Read the model definition and answer for the solid it produces. Units are mm, in the model's axes. Give positions to 0.01 mm unless a question says otherwise; leave off trailing zeros. Write each loop counter-clockwise with the first axis right and the second up, starting at its lowest first coordinate (ties: lowest second). Pieces come first, ordered by that corner, then holes. Notation, with made-up numbers: (34, 24) -> (93, 24) arc R34 cw to (93, 58) -> close; hole circle Ø3 at (38, 51). An arc over 180 degrees is marked (long way). Use a Markdown table: item, result.
from build123d import *

# Parameters (mm, degrees)
SKETCH1_R      = 7.9375
EXTRUDE1_DEPTH = 78.8
SKETCH2_R      = 3.175
CHAMFER1_SIZE  = 1


with BuildPart() as part:
    # Sketch1 → Extrude1 (new body)
    with BuildSketch(Plane(origin=(0, 0, 0), x_dir=(0, 0, -1), z_dir=(1, 0, 0))):
        Circle(SKETCH1_R)
    extrude(amount=EXTRUDE1_DEPTH)

    # Sketch2 → Cut-Revolve1 (revolve, cut)
    with BuildSketch(Plane(origin=(0, 0, 0), x_dir=(1, 0, 0), z_dir=(0, 1, 0))):
        with Locations((69.8, 9.525)):
            Circle(SKETCH2_R)
    revolve(axis=Axis((0, 0, 0), (1, 0, 0)), mode=Mode.SUBTRACT)

    # Chamfer1
    chamfer1_edges = [part.edges().sort_by_distance(p)[0] for p in [
        (78.8, 0, 7.9375),
    ]]
    chamfer(chamfer1_edges, length=CHAMFER1_SIZE)


solid = part.part
Item 1: Each of these flat-tipped pins is pushed along its axis until it touches: P1, Ø1, axis at x = 31, y = 3.5, coming from the -Z side; P2, Ø1.5, axis at y = -0.5, z = 1, coming from the -X side; P3, Ø8, axis at x = 40, y = -6, coming from the -Z side; P4, Ø1.5, axis at x = 16.5, z = -5, coming from the -Y side. Where does it stop, or does it pass through?
Return value:
| item | result |
|---|---|
| P1 | z = -7.35 |
| P2 | x = 0 |
| P3 | z = -7.68 |
| P4 | y = -6.7 |
Item 2: Straight lines are drawn through the part: line 1 along Y through (x, z) = (65, 0.5); line 2 along X through (y, z) = (-3.5, 7). For each, find the intervals that lie inside material, in ascending order. Write a range as [from, to].
Return value:
| item | result |
|---|---|
| line 1 | [-7.92, 7.92] |
| line 2 | [0, 67.12], [72.48, 77.91] |
Item 3: A cutting plane is placed at A-A (x = 38). Give the vertices of the cut face in (y, z) (1 decimal), then the cut area to 3 significant figures.
Return value:
| item | result |
|---|---|
| outline | circle Ø15.9 at (0, 0) |
| area | 198 mm^2 |
